```python
from build123d import *

# Parameters (mm, degrees)
F0_R     = 10.5
F0_W     = 22.3368
F0_H     = 5.842
F0_W_2   = 5.842
F0_H_2   = 22.337
F0_H_3   = 22.3366
F0_W_3   = 22.337
F0_W_4   = 22.3366
F1_DEPTH = 5.842


with BuildPart() as f1:
    # F0 (on Right) → F1 (new body)
    with BuildSketch(Plane.YZ):
        Polygon((-33.5052, 50), (-50, 50), (-50, 33.5052), (-50, 11.1682), (-50, -11.1686), (-50, -33.5052), (-50, -50), (-33.5052, -50), (-11.1682, -50), (11.1686, -50), (33.5052, -50), (50, -50), (50, -33.5052), (50, -11.1686), (50, 11.1682), (50, 33.5052), (50, 50), (33.5052, 50), (11.1684, 50), (-11.1684, 50), align=None)
        with Locations((-34.085574, -34.319336)):
            Circle(F0_R, mode=Mode.SUBTRACT)
        with Locations((-22.3368, 52.921)):
            Rectangle(F0_W, F0_H)
        with Locations((-52.921, 22.3367)):
            Rectangle(F0_W_2, F0_H_2)
        with Locations((22.3368, 52.921)):
            Rectangle(F0_W, F0_H)
        with Locations((-52.921, -22.3369)):
            Rectangle(F0_W_2, F0_H_3)
        with Locations((52.921, 22.3367)):
            Rectangle(F0_W_2, F0_H_2)
        with Locations((-22.3367, -52.921)):
            Rectangle(F0_W_3, F0_H)
        with Locations((52.921, -22.3369)):
            Rectangle(F0_W_2, F0_H_3)
        with Locations((22.3369, -52.921)):
            Rectangle(F0_W_4, F0_H)
    extrude(amount=F1_DEPTH)


solid = f1.part
```
Design review of the part built by this model. Coordinates are the model's own, in mm. A direction names the side the tool comes from. Coordinates: 2 decimals unless noted, no trailing zeros. Order: outer loops, then holes, each group sorted by start corner. A loop starts at its lowest first (then second) coordinate and runs counter-clockwise, first axis right, second up. Notation, with made-up numbers: (85, 55.25) -> (113, 55.25) arc R26 cw to (113, 70.25) -> close; hole circle Ø5 at (86, 32). An arc over 180 degrees is marked (long way). One line per item, written item: value. Start each with the question number.
Q1. Insertion check: pin 1 Ø3 at (x, z) = (2.5, 39) entering from -Y; pin 2 Ø1.8 at (x, y) = (4, -2) entering from +Z; pin 3 Ø1 at (x, z) = (1, 38.5) entering from +Y. Each pin has a flat end and moves straight along its axis. Give the tip position at first contact, or say it passes through.
Q2. Tool access review of faces 4 (the flat face through (3, -50, 42)), 5 (the flat face through (3, 53, 33.505)), 6 (the flat face through (3, 50, 0)), 7 (the flat face through (3, -33.505, -53)): name each direction out of +Z, -Z, +X, -X, +Y, -Y from which nothing blocks a thin tool from reaching the whole face with its end or side.
Q3. Mouldability with a two-part tool opening along Z and no side actions: class faces 1 (the flat face through (3, 53, 11.168)), 2 (the flat face through (3, -53, 33.505)), 3 (the flat face through (3, -42, -50)) as pulls with the +Z half, pulls with the -Z half, needs draft (parallel to the pull), parting line crosses it, or undercut.
Q4. For probe 1 along Y at (x, z) = (5.15, -10); probe 2 along Z at (x, y) = (1.35, -31); probe 3 along Z at (x, y) = (5.05, -40), list the stretches that pass through material, from the lowest coordinate up.
Q5. Take a section at B-B, the plane y = -7. State the section outline as (x, z) points.
Q6. Take a section at A-A, the plane z = -39. State the section outline as (x, y) points, then the cut area to 3 significant figures.
Values follow:
1. pin 1: stops at y = -50
1. pin 2: stops at z = 50
1. pin 3: stops at y = 50
2. face 4: +Z, +X, -X, -Y
2. face 5: +Z, +X, -X, +Y
2. face 6: +X, -X, +Y
2. face 7: -Z, +X, -X, -Y
3. face 1: undercut
3. face 2: pulls with the +Z half
3. face 3: pulls with the -Z half
4. probe 1: y = -50 to 50
4. probe 2: z = -55.84 to -44.36, -24.28 to 55.84
4. probe 3: z = -50 to -43, -25.64 to 50
5. outline: (0, -50) -> (5.84, -50) -> (5.84, 50) -> (0, 50) -> close
6. outline: (0, -50) -> (5.84, -50) -> (5.84, -43.48) -> (0, -43.48) -> close; (0, -24.69) -> (5.84, -24.69) -> (5.84, 50) -> (0, 50) -> close
6. area: 474 mm2
